Print and shaded views of the part. All mm, measured from the part's lowest x, y and z. Give positions to 0.01 mm unless a question says otherwise; leave off trailing zeros. Loops run counter-clockwise (first coordinate to the right, second up) from the corner with the lowest first, then second, coordinate; pieces in that order, holes last. Notation, with made-up numbers: (15, -15.5) -> (23, -15.5) arc R10 ccw to (23, 0.5) -> close; hole circle Ø5 at (50, 85). An arc over 180 degrees is marked (long way). Answer as a JSON object with one key per item and string values. Group by question number.
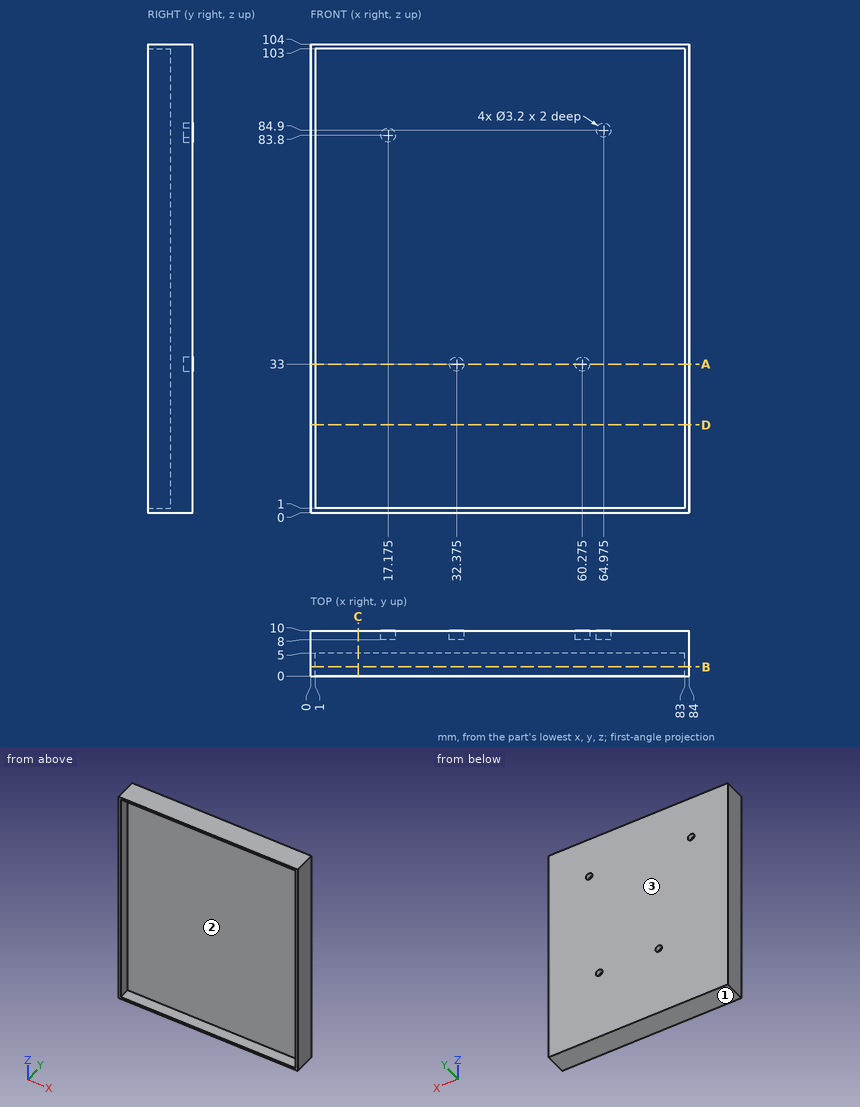
(1) Saw through at B-B on y = 2. List the corners of the cut face in (x, z), plus the area to 3 significant figures.
(2) Saw through at A-A on z = 33. List the corners of the cut face in (x, y) (3 decimals), plus the area to 3 significant figures.
(3) Probe line 1 along X through (y, z) = (1.25, 91); line 2 along X through (y, z) = (9.05, 84.9) (3 decimals); line 3 along Z through (x, y) = (14.5, 2.5). List the from-to ranges inside material, lowest first. Write a range as [from, to].
(4) Pull direction Z, two halves, no side cores. Call the marked faces 1, 2 and 3: pulls with the +Z half, pulls with the -Z half, needs draft (parallel to the pull), parting line crosses it, or undercut.
(5) Saw through at D-D on z = 19.5. List the corners of the cut face in (x, y).
(6) Pin check, flat tips, straight feed: pin 1 (2.5 mm diameter, centred on x = 16.5, z = 84.5, fed in from +Y); pin 2 (2.5 mm diameter, centred on x = 32.375, z = 33, fed in from +Y); pin 3 (1.9 mm diameter, centred on x = 60.275, z = 33, fed in from -Y). Stop position of each tip, or through.
(7) Saw through at C-C on x = 10.5. List the corners of the cut face in (y, z).
Calculated:
{
 "1": {"outline": "(0, 0) -> (84, 0) -> (84, 104) -> (0, 104) -> close; hole (1, 1) -> (83, 1) -> (83, 103) -> (1, 103) -> close", "area": "372 mm^2"},
 "2": {"outline": "(0, 0) -> (1, 0) -> (1, 5) -> (83, 5) -> (83, 0) -> (84, 0) -> (84, 10) -> (61.875, 10) -> (61.875, 8) -> (58.675, 8) -> (58.675, 10) -> (33.975, 10) -> (33.975, 8) -> (30.775, 8) -> (30.775, 10) -> (0, 10) -> close", "area": "417 mm^2"},
 "3": {"line 1": "x = [0, 1], [83, 84]", "line 2": "x = [0, 16.013], [18.337, 63.375], [66.575, 84]", "line 3": "z = [0, 1], [103, 104]"},
 "4": {"face 1": "pulls with the -Z half", "face 2": "undercut", "face 3": "needs draft"},
 "5": {"outline": "(0, 0) -> (1, 0) -> (1, 5) -> (83, 5) -> (83, 0) -> (84, 0) -> (84, 10) -> (0, 10) -> close"},
 "6": {"pin 1": "stops at y = 10", "pin 2": "stops at y = 8", "pin 3": "stops at y = 5"},
 "7": {"outline": "(0, 0) -> (10, 0) -> (10, 104) -> (0, 104) -> (0, 103) -> (5, 103) -> (5, 1) -> (0, 1) -> close"}
}
